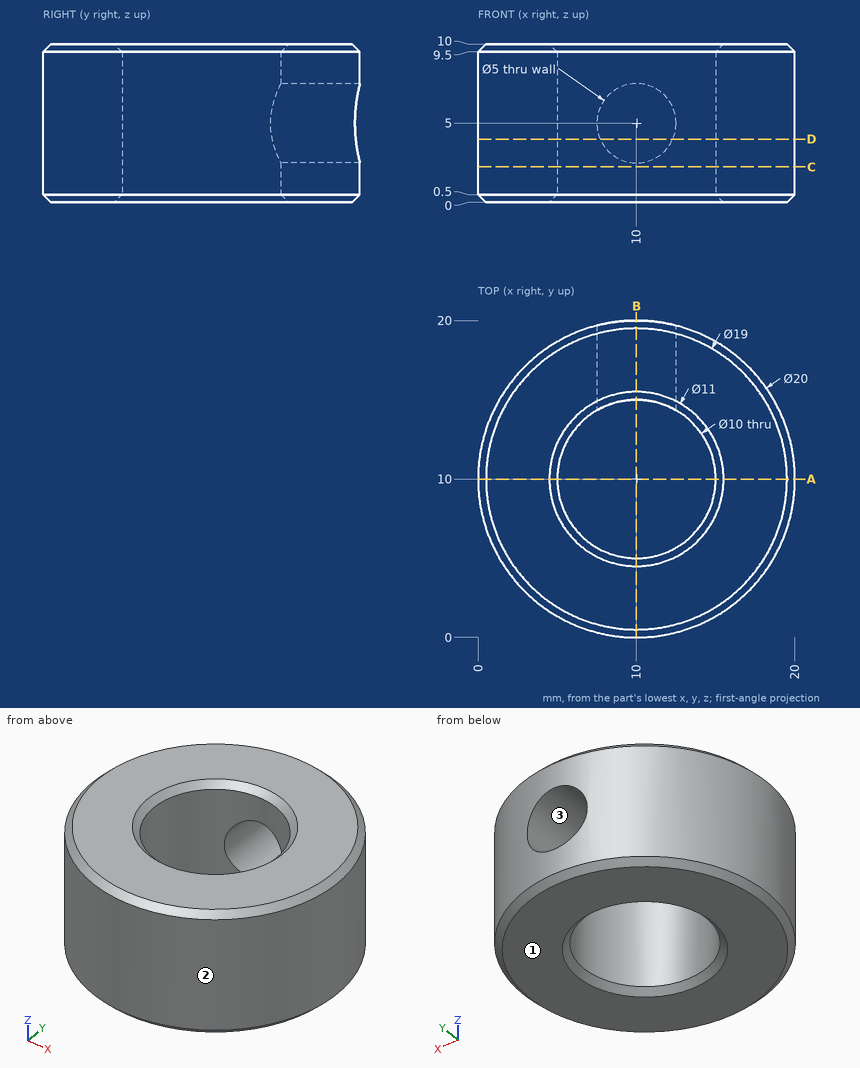
Could you check a few things on this drawing? It's one solid part, dimensions in mm from its lowest x, y, z. Coordinates: 2 decimals unless noted, no trailing zeros. Write each loop counter-clockwise with the first axis right and the second up, starting at its lowest first coordinate (ties: lowest second). Pieces come first, ordered by that corner, then holes. Notation, with made-up numbers: (79.25, 79.5) - (119.25, 79.5) arc R9 cw to (119.25, 91.5) - close; hole circle Ø11 at (-18, -7). An arc over 180 degrees is marked (long way). Return JSON: item names as keys, results as strings. Group by question number.
Item 1: Please list where these lines run through material, in increasing order: probe 1 along X at (y, z) = (10.25, 9); probe 2 along Z at (x, y) = (10, 15.9); probe 3 along X at (y, z) = (9, 8).
Item 2: If we section it at C-C (z = 2.25): Write out the boundary of the cut face in (x, y).
Item 3: If we section it at B-B (x = 10): Write out the boundary of the cut face in (y, z).
Item 4: I'm going to push flat-ended pins straight in: pin 1 Ø2 at (x, z) = (13.5, 2) entering from +Y; pin 2 Ø1 at (x, z) = (17.5, 4) entering from -Y; pin 3 Ø5 at (x, z) = (2.5, 8.5) entering from -Y; pin 4 Ø5 at (x, y) = (17.5, 4) entering from +Z. Where does each tip first touch, or does it pass through?
Item 5: If we section it at D-D (z = 4): Write out the boundary of the cut face in (x, y).
Item 6: We'd pull the mould along X, two halves only. Please class the marked faces 1, 2 and 3: pulls with the +X half, pulls with the -X half, needs draft (parallel to the pull), parting line crosses it, or undercut.
Item 7: If we section it at A-A (y = 10): Write out the boundary of the cut face in (x, z).
Return value:
{
 "1": {"probe 1": "x = 0 to 5.01, 14.99 to 20", "probe 2": "z = 0 to 2.5, 7.5 to 10", "probe 3": "x = 0.05 to 5.1, 14.9 to 19.95"},
 "2": {"outline": "circle Ø20 at (10, 10); hole circle Ø10 at (10, 10)"},
 "3": {"outline": "(0, 0.5) - (0.5, 0) - (4.5, 0) - (5, 0.5) - (5, 9.5) - (4.5, 10) - (0.5, 10) - (0, 9.5) - close; (15, 0.5) - (15.5, 0) - (19.5, 0) - (20, 0.5) - (20, 2.5) - (15, 2.5) - close; (15, 7.5) - (20, 7.5) - (20, 9.5) - (19.5, 10) - (15.5, 10) - (15, 9.5) - close"},
 "4": {"pin 1": "stops at y = 19.68", "pin 2": "stops at y = 2.86", "pin 3": "stops at y = 1.34", "pin 4": "stops at z = 10"},
 "5": {"outline": "(7.71, 14.44) - (7.71, 19.73) arc R10 ccw (long way) to (12.29, 19.73) - (12.29, 14.44) arc R5 cw (long way) to start"},
 "6": {"face 1": "needs draft", "face 2": "parting line crosses it", "face 3": "undercut"},
 "7": {"outline": "(0, 0.5) - (0.5, 0) - (4.5, 0) - (5, 0.5) - (5, 9.5) - (4.5, 10) - (0.5, 10) - (0, 9.5) - close; (15, 0.5) - (15.5, 0) - (19.5, 0) - (20, 0.5) - (20, 9.5) - (19.5, 10) - (15.5, 10) - (15, 9.5) - close"}
}
